The listing builds one solid part. Answer for the finished solid, in the listing's coordinates (mm). Coordinates: 2 decimals unless noted, no trailing zeros. Order: outer loops, then holes, each group sorted by start corner. A loop starts at its lowest first (then second) coordinate and runs counter-clockwise, first axis right, second up. Notation, with made-up numbers: (74, 5.25) -> (86, 5.25) arc R26 cw to (86, 32.25) -> close; hole circle Ø9 at (-17.5, 31.5). An arc over 180 degrees is marked (long way). Return JSON: item names as keys, results as strings.
Autodesk Inventor part; units mm, degrees
ref_plane "YZ Plane" through (0, 0, 0) normal (1, 0, 0) x (0, 1, 0)
ref_plane "XZ Plane" through (0, 0, 0) normal (0, 1, 0) x (-1, 0, 0)
ref_plane "XY Plane" through (0, 0, 0) normal (0, 0, 1) x (1, 0, 0)
sketch "Sketch1" plane through (0, 0, 0) normal (0, 1, 0) x (-1, 0, 0)
  line L0 (-12.7, 8) -> (8, 8)
  line L1 (8, 8) -> (-12.7, 8)
  line L2 (8, 8) -> (8, -29.85)
  line L3 (8, 8) -> (8, -29.85)
  line L4 (-38.6, -29.85) -> (-38.6, -21.85)
  line L5 (8, -29.85) -> (-38.6, -29.85)
  line L6 (-38.6, -2.35) -> (-38.6, -21.85)
  line L7 (-38.6, -29.85) -> (-38.6, -2.35)
  line L8 (-94.4, -2.35) -> (-38.6, -2.35)
  line L9 (-38.6, -2.35) -> (-94.4, -2.35)
  line L10 (-94.4, -21.85) -> (-94.4, -29.85)
  line L11 (-94.4, -2.35) -> (-94.4, -29.85)
  line L12 (-94.4, -29.85) -> (-160, -29.85)
  line L13 (-94.4, -29.85) -> (-160, -29.85)
  line L14 (-160, -29.85) -> (-160, 8)
  line L15 (-160, -29.85) -> (-160, 8)
  line L16 (-139.3, 8) -> (-139.3, 51.15)
  line L17 (-160, 8) -> (-139.3, 8)
  line L18 (-139.3, 8) -> (-139.3, 51.15)
  line L19 (-139.3, 51.15) -> (-12.7, 51.15)
  line L20 (-139.3, 51.15) -> (-12.7, 51.15)
  line L21 (-12.7, 51.15) -> (-12.7, 8)
  line L22 (-12.7, 51.15) -> (-12.7, 8)
  circle A0 centre (-34.6, -25.85) radius 1.875
  circle A1 centre (-34.6, -25.85) radius 1.55
  circle A2 centre (4, 4) radius 1.55
  circle A3 centre (-76, 47.15) radius 1.55
  circle A4 centre (-156, 4) radius 1.55
  circle A5 centre (-98.4, -25.85) radius 1.55
  point P0 (0, 0)
  dimension "d2" = 3.1
extrude "Extrusion1" add sketch "Sketch1" along normal blind 1.5 contours L0 L2 L5 L4 L6 L8 L11 L10 L12 L14 L17 L16 L19 L21 | A0
sketch "Sketch2" plane through (0, 0, 0) normal (0, -1, 0) x (1, 0, 0)
  line L0 (12.7, 8) -> (12.7, 51.15)
  circle A0 centre (12.7, 51.15) radius 4
  line L1 (12.7, 51.15) -> (139.3, 51.15)
  circle A1 centre (139.3, 51.15) radius 4
  line L2 (160, 8) -> (160, -29.85)
  circle A2 centre (160, 8) radius 4
  circle A3 centre (160, -29.85) radius 4
  circle A4 centre (94.4, -29.85) radius 4
  circle A5 centre (38.4923, -29.85) radius 4
  line L3 (38.6, -29.85) -> (-8, -29.85)
  circle A6 centre (-8, -29.85) radius 4
  circle A7 centre (-8, 8) radius 4
  point P0 (0, 0)
  dimension "d7" = 8
  dimension "d8" = 8
  dimension "d9" = 8
  dimension "d10" = 8
  dimension "d11" = 8
  dimension "d12" = 8
  dimension "d13" = 8
  dimension "d14" = 8
extrude "Extrusion2" add sketch "Sketch2" against normal blind 0.2
properties part number "TopPlate"
1. The part is cut by section A-A on y = 0.5. Give the vertices of the cut face in (x, z), and give its area (3 significant figures).
Answer block:
{"outline": "(-8, -29.85) -> (38.6, -29.85) -> (38.6, -2.35) -> (94.4, -2.35) -> (94.4, -29.85) -> (160, -29.85) -> (160, 8) -> (139.3, 8) -> (139.3, 51.15) -> (12.7, 51.15) -> (12.7, 8) -> (-8, 8) -> close; hole circle Ø3.1 at (-4, 4); hole circle Ø3.1 at (34.6, -25.85); hole circle Ø3.1 at (76, 47.15); hole circle Ø3.1 at (98.4, -25.85); hole circle Ø3.1 at (156, 4)", "area": "10,200 mm2"}
2. Each of these flat-tipped pins is pushed along its axis until it touches: pin 1 Ø1.9 at (x, z) = (34.6, -25.85) entering from -Y; pin 2 Ø4 at (x, z) = (11, 53) entering from +Y; pin 3 Ø0.8 at (y, z) = (0.5, 39.5) entering from +X. Where does it stop, or does it pass through?
Answer block:
{"pin 1": "passes through", "pin 2": "stops at y = 0.2", "pin 3": "stops at x = 139.3"}
3. Consider line 1 (X direction, y = 1.05, z = -18); line 2 (Z direction, x = 156, y = 0.8); line 3 (Z direction, x = 34.6, y = 0.5). Determine where each line is inside the solid, lowest interval first. Write a range as from..to.
Answer block:
{"line 1": "x = -8..38.6, 94.4..160", "line 2": "z = -29.85..2.45, 5.55..8", "line 3": "z = -29.85..-27.4, -24.3..51.15"}
4. The part is cut by section C-C on z = 37. Give the vertices of the cut face in (x, y), and give its area (3 significant figures).
Answer block:
{"outline": "(12.7, 0) -> (139.3, 0) -> (139.3, 1.5) -> (12.7, 1.5) -> close", "area": "190 mm2"}
5. Determine the mould class of faces 1 (the face through (13, 0.2, 52)), 2 (the face through (39, 0.2, -31)) for opening direction X: pulls with the +X half, pulls with the -X half, needs draft (parallel to the pull), parting line crosses it, or undercut.
Answer block:
{"face 1": "needs draft", "face 2": "undercut"}
6. The part is cut by section B-B on x = 117.5. Give the vertices of the cut face in (y, z), and give its area (4 significant figures).
Answer block:
{"outline": "(0, -29.85) -> (1.5, -29.85) -> (1.5, 51.15) -> (0, 51.15) -> close", "area": "121.5 mm2"}
